The drawing under review shows one solid part. Ordinate dimensions are in mm from its lowest x, y, z. A direction names the side the tool comes from. Coordinates: 2 decimals unless noted, no trailing zeros. Write each loop counter-clockwise with the first axis right and the second up, starting at its lowest first coordinate (ties: lowest second). Pieces come first, ordered by that corner, then holes.
1) We need section A-A on x = 37.5. Write out the cut boundary in (y, z).
2) We need section C-C on y = 17. Write out the cut boundary in (x, z) (1 decimal).
3) We need section D-D on z = 10.5. Write out the cut boundary in (x, y) (1 decimal), then the cut area to 3 significant figures.
4) Insertion check: P1, Ø11, axis at y = 42, z = 48.5, coming from the -X side; P2, Ø18, axis at x = 48, z = 22.5, coming from the -Y side; P3, Ø11, axis at x = 67.5, y = 40.5, coming from the +Z side; P4, Ø8, axis at y = 41, z = 40, coming from the +X side. Each pin has a flat end and moves straight along its axis. Give the tip position at first contact, or say it passes through.
5) To check wall thickness, follow line 1 along Y through (x, z) = (37.5, 58); line 2 along Y through (x, z) = (37, 57) (1 decimal); line 3 along Z through (x, y) = (7.5, 39.5). State the ranges of each line that lie inside material, in increasing order.
6) Mouldability with a two-part tool opening along Z and no side actions: class the marked faces 4, 5 and 6 as pulls with the +Z half, pulls with the -Z half, needs draft (parallel to the pull), parting line crosses it, or undercut.
7) For the marked faces 1, 2 and 3, list the 3-axis set-ups (+Z, -Z, +X, -X, +Y, -Y) from which the entire face can be reached by the end or side of a thin tool; tool diameter is ignored.
8) We need section B-B on x = 7.5. Write out the cut boundary in (y, z), then the cut area to 3 significant figures.
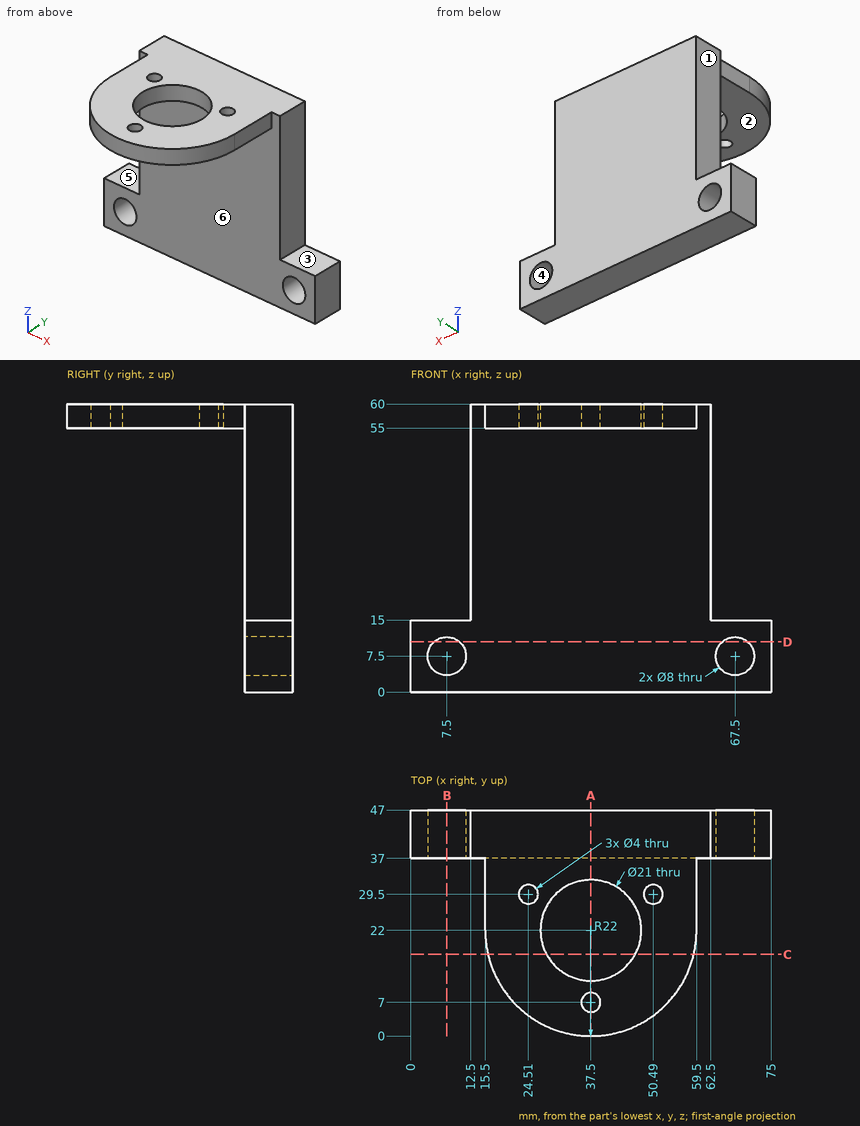
Result:
1. outline: (0, 55) - (5, 55) - (5, 60) - (0, 60) - close; (9, 55) - (11.5, 55) - (11.5, 60) - (9, 60) - close; (32.5, 55) - (37, 55) - (37, 0) - (47, 0) - (47, 60) - (32.5, 60) - close
2. outline: (16.1, 55) - (28.3, 55) - (28.3, 60) - (16.1, 60) - close; (46.7, 55) - (58.9, 55) - (58.9, 60) - (46.7, 60) - close
3. outline: (0, 37) - (4.9, 37) - (4.9, 47) - (0, 47) - close; (10.1, 37) - (64.9, 37) - (64.9, 47) - (10.1, 47) - close; (70.1, 37) - (75, 37) - (75, 47) - (70.1, 47) - close
3. area: 644 mm2
4. P1: stops at x = 12.5
4. P2: stops at y = 37
4. P3: stops at z = 60
4. P4: stops at x = 62.5
5. line 1: y = 0 to 5, 9 to 11.5, 32.5 to 47
5. line 2: y = 0 to 5.1, 8.9 to 11.5, 32.5 to 47
5. line 3: z = 0 to 3.5, 11.5 to 15
6. face 4: undercut
6. face 5: pulls with the +Z half
6. face 6: needs draft
7. face 1: +Z, -X, +Y, -Y
7. face 2: -Z, +X, -X, -Y
7. face 3: +Z, +X, +Y, -Y
8. outline: (37, 0) - (47, 0) - (47, 3.5) - (37, 3.5) - close; (37, 11.5) - (47, 11.5) - (47, 15) - (37, 15) - close
8. area: 70.0 mm2
